Design review of the part built by this model. Coordinates are the model's own, in mm. Give positions to 0.01 mm unless a question says otherwise; leave off trailing zeros. Write each loop counter-clockwise with the first axis right and the second up, starting at its lowest first coordinate (ties: lowest second). Pieces come first, ordered by that corner, then holes. Notation, with made-up numbers: (47.5, 33) -> (73.5, 33) arc R36 ccw to (73.5, 71) -> close; hole circle Ø1 at (52, 81). An arc over 180 degrees is marked (long way). Return JSON: item names as keys, results as strings. Group by question number.
from build123d import *

# Parameters (mm, degrees)
BOSS_EXTRUDE1_DEPTH      = 431.8
BOSS_EXTRUDE1_DEPTH_BACK = 304.8
SKETCH1_W                = 63.5
SKETCH1_H                = 63.5
SKETCH1_W_2              = 58.7375
SKETCH1_H_2              = 58.7375
SKETCH2_R                = 25.4
CUT_EXTRUDE1_DEPTH       = 438.597477712


with BuildPart() as part:
    # Sketch1 → Boss-Extrude1 (new, two sides: drawn at the far end of the back side and taken through both)
    with BuildSketch(Plane.XY.offset(-BOSS_EXTRUDE1_DEPTH_BACK)):
        Rectangle(SKETCH1_W, SKETCH1_H)
        Rectangle(SKETCH1_W_2, SKETCH1_H_2, mode=Mode.SUBTRACT)
    extrude(amount=BOSS_EXTRUDE1_DEPTH + BOSS_EXTRUDE1_DEPTH_BACK)

    # Sketch2 → Cut-Extrude1 (cut, through all)
    with BuildSketch(Plane.ZY.offset(31.75)):
        with Locations((-254, 0)):
            Circle(SKETCH2_R)
        with Locations((203.2, 0)):
            Circle(SKETCH2_R)
    extrude(amount=-CUT_EXTRUDE1_DEPTH, mode=Mode.SUBTRACT)


solid = part.part
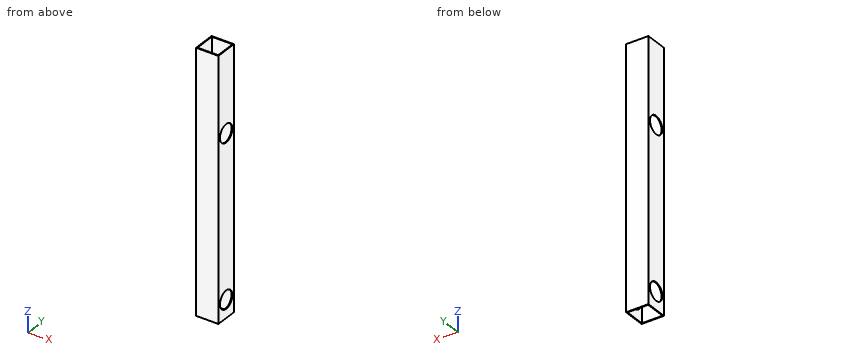
Q1. For L1, parallel to Y at x = -10, z = 295.5; L2, parallel to Y at x = 30.2, z = -254, list the stretches that pass through material, from the lowest coordinate up. Write a range as from..to.
Q2. Take a section at C-C, the plane x = -5. Give the boundary of the cut face in (y, z), plus the area to 3 significant figures.
Q3. Take a section at B-B, the plane z = 27. Give the boundary of the cut face in (x, y), plus the area to 3 significant figures.
Q4. Insertion check: pin 1 (8 mm diameter, centred on y = 20.5, z = 210, fed in from +X). The pin has a flat end and moves straight along its axis. Give the tip position at first contact, or say it passes through.
Q5. Take a section at A-A, the plane y = 0. Give the boundary of the cut face in (x, z).
Q6. Take a section at D-D, the plane z = 203.2. Give the boundary of the cut face in (x, y), plus the area to 3 significant figures.
Final values:
{
 "1": {"L1": "y = -31.75..-29.37, 29.37..31.75", "L2": "y = -31.75..-25.4, 25.4..31.75"},
 "2": {"outline": "(-31.75, -304.8) -> (-29.37, -304.8) -> (-29.37, 431.8) -> (-31.75, 431.8) -> close; (29.37, -304.8) -> (31.75, -304.8) -> (31.75, 431.8) -> (29.37, 431.8) -> close", "area": "3,510 mm²"},
 "3": {"outline": "(-31.75, -31.75) -> (31.75, -31.75) -> (31.75, 31.75) -> (-31.75, 31.75) -> close; hole (-29.37, -29.37) -> (29.37, -29.37) -> (29.37, 29.37) -> (-29.37, 29.37) -> close", "area": "582 mm²"},
 "4": {"pin 1": "stops at x = 31.75"},
 "5": {"outline": "(-31.75, -304.8) -> (-29.37, -304.8) -> (-29.37, -279.4) -> (-31.75, -279.4) -> close; (-31.75, -228.6) -> (-29.37, -228.6) -> (-29.37, 177.8) -> (-31.75, 177.8) -> close; (-31.75, 228.6) -> (-29.37, 228.6) -> (-29.37, 431.8) -> (-31.75, 431.8) -> close; (29.37, -304.8) -> (31.75, -304.8) -> (31.75, -279.4) -> (29.37, -279.4) -> close; (29.37, -228.6) -> (31.75, -228.6) -> (31.75, 177.8) -> (29.37, 177.8) -> close; (29.37, 228.6) -> (31.75, 228.6) -> (31.75, 431.8) -> (29.37, 431.8) -> close"},
 "6": {"outline": "(-31.75, -31.75) -> (31.75, -31.75) -> (31.75, -25.4) -> (29.37, -25.4) -> (29.37, -29.37) -> (-29.37, -29.37) -> (-29.37, -25.4) -> (-31.75, -25.4) -> close; (-31.75, 25.4) -> (-29.37, 25.4) -> (-29.37, 29.37) -> (29.37, 29.37) -> (29.37, 25.4) -> (31.75, 25.4) -> (31.75, 31.75) -> (-31.75, 31.75) -> close", "area": "340 mm²"}
}
